Answer from the drawing. Dimensions are ordinates in mm from the lowest x, y and z of the part. Coordinates: 2 decimals unless noted, no trailing zeros. Write each loop counter-clockwise with the first axis right and the second up, starting at its lowest first coordinate (ties: lowest second). Pieces come first, ordered by that corner, then holes.
1) Find the intervals of material crossed by line 1 (X direction, y = 3.25, z = 14.98); line 2 (X direction, y = 4, z = 35); line 3 (Z direction, x = 59, y = 5.75), in increasing order.
2) The part is cut by section A-A (z = 35). Determine the outline of the cut face in (x, y).
3) The part is cut by section D-D (y = 3.25). Determine the outline of the cut face in (x, z), then the cut area to 3 significant figures.
4) The part is cut by section C-C (z = 14.98). Determine the outline of the cut face in (x, y), then the cut area to 3 significant figures.
5) This flat-tipped pin is pushed along its axis until it touches: pin 1 Ø20.5 at (x, z) = (50, 35) entering from -Y. Where does it stop, or does it pass through?
6) The part is cut by section B-B (x = 50). Determine the outline of the cut face in (y, z).
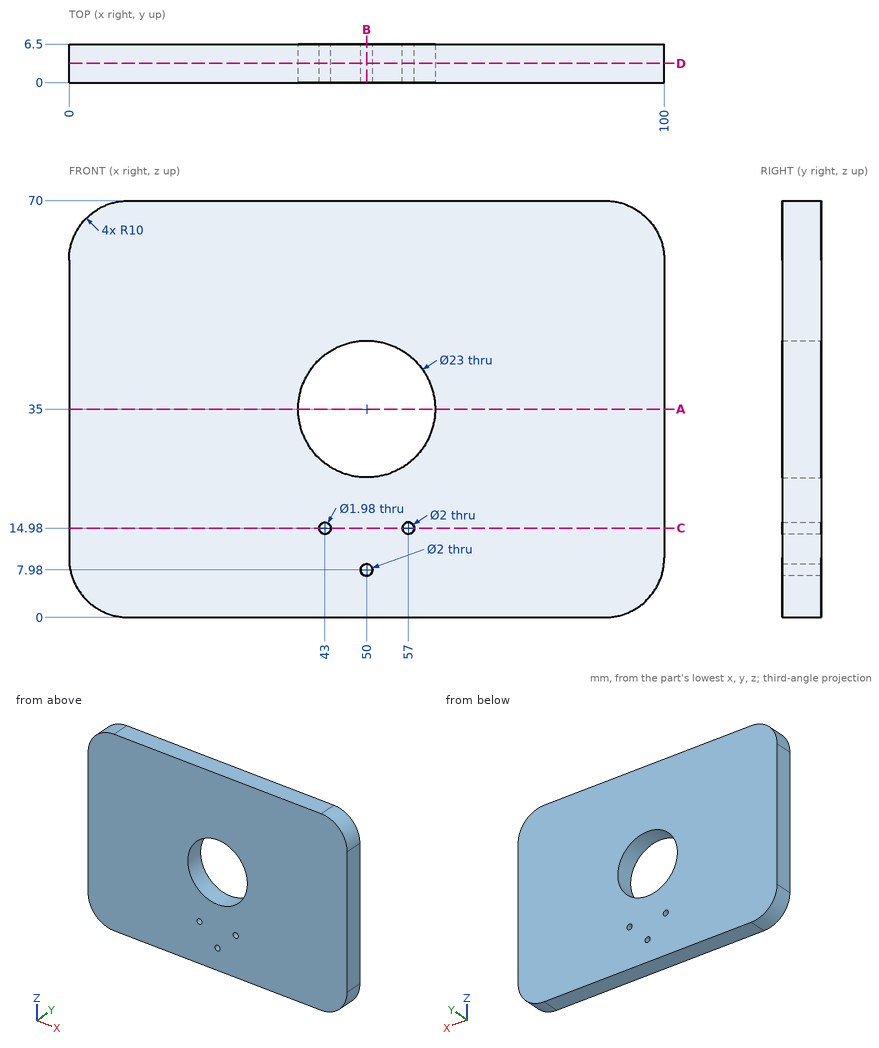
Reported:
1. line 1: x = 0 to 42.01, 43.99 to 56, 58 to 100
1. line 2: x = 0 to 38.5, 61.5 to 100
1. line 3: z = 0 to 27.84, 42.16 to 70
2. outline: (0, 0) - (38.5, 0) - (38.5, 6.5) - (0, 6.5) - close; (61.5, 0) - (100, 0) - (100, 6.5) - (61.5, 6.5) - close
3. outline: (0, 10) arc R10 ccw to (10, 0) - (90, 0) arc R10 ccw to (100, 10) - (100, 60) arc R10 ccw to (90, 70) - (10, 70) arc R10 ccw to (0, 60) - close; hole circle Ø23 at (50, 35); hole circle Ø1.98 at (43, 14.98); hole circle Ø2 at (50, 7.98); hole circle Ø2 at (57, 14.98)
3. area: 6,490 mm2
4. outline: (0, 0) - (42.01, 0) - (42.01, 6.5) - (0, 6.5) - close; (43.99, 0) - (56, 0) - (56, 6.5) - (43.99, 6.5) - close; (58, 0) - (100, 0) - (100, 6.5) - (58, 6.5) - close
4. area: 624 mm2
5. pin 1: passes through
6. outline: (0, 0) - (6.5, 0) - (6.5, 6.98) - (0, 6.98) - close; (0, 8.98) - (6.5, 8.98) - (6.5, 23.5) - (0, 23.5) - close; (0, 46.5) - (6.5, 46.5) - (6.5, 70) - (0, 70) - close
